Verification items for the finished model (mm, model axes). Give positions to 0.01 mm unless a question says otherwise; leave off trailing zeros. Write each loop counter-clockwise with the first axis right and the second up, starting at its lowest first coordinate (ties: lowest second). Pieces come first, ordered by that corner, then holes. Notation, with made-up numbers: (62, -23) - (83, -23) arc R21 ccw to (83, -6) - close; hole circle Ø10 at (32.25, 76). An arc over 180 degrees is marked (long way). Put each result on its own line as item: value.
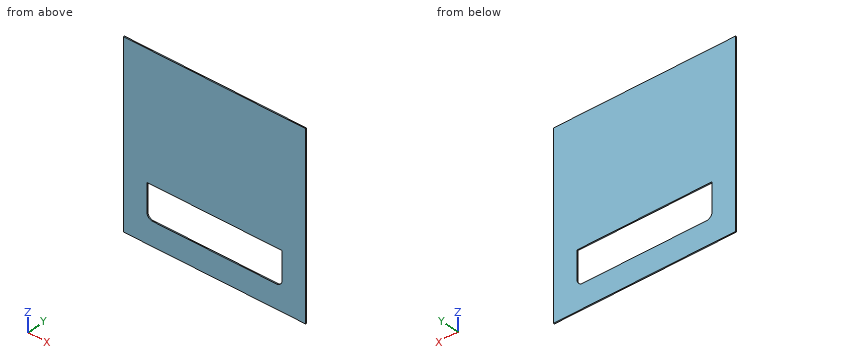
from build123d import *

# Parameters (mm, degrees)
SKETCH_1_W          = 162
SKETCH_1_H          = 162
EXTRUDE_1_DEPTH     = 1
CUT_EXTRUDE_1_REACH = 3
SKETCH_2_W          = 120
SKETCH_2_H          = 30
FILLET_1_R          = 5


with BuildPart() as part:
    # 草图1 → 凸台-拉伸1 (new body)
    with BuildSketch(Plane(origin=(0, 0, 0), x_dir=(1, 0, 0), z_dir=(0, 1, 0))):
        Rectangle(SKETCH_1_W, SKETCH_1_H)
    extrude(amount=EXTRUDE_1_DEPTH)

    # 草图2 → 切除-拉伸1 (cut, up to next)
    with BuildSketch(Plane.XZ, mode=Mode.PRIVATE) as cut_extrude_1_sk1:
        with Locations((0, -45)):
            Rectangle(SKETCH_2_W, SKETCH_2_H)
    cut_extrude_1_tool1 = extrude(cut_extrude_1_sk1.sketch, amount=-CUT_EXTRUDE_1_REACH, mode=Mode.PRIVATE) & part.part
    add(cut_extrude_1_tool1.solids().sort_by_distance((0, 0, -45))[0], mode=Mode.SUBTRACT)

    # 圆角1
    fillet_1_edges = [part.edges().sort_by_distance(p)[0] for p in [
        (60, 0.5, -60),
        (-60, 0.5, -60),
    ]]
    fillet(fillet_1_edges, radius=FILLET_1_R)


solid = part.part
Q1. Go/stop test with a flat-tipped pin: pin 1 Ø3 at (x, z) = (54.5, 31) entering from -Y. Record where the tip stops, or that it passes through.
Answers follow:
pin 1: stops at y = 0
Q2. Section check C-C, the plane y = 0.3. Record the cut outline in (x, z).
Answers follow:
outline: (-81, -81) - (81, -81) - (81, 81) - (-81, 81) - close; hole (-60, -55) arc R5 ccw to (-55, -60) - (55, -60) arc R5 ccw to (60, -55) - (60, -30) - (-60, -30) - close
Q3. Section check A-A, the plane x = 6. Record the cut outline in (y, z).
Answers follow:
outline: (0, -81) - (1, -81) - (1, -60) - (0, -60) - close; (0, -30) - (1, -30) - (1, 81) - (0, 81) - close
Q4. Scan lines: line 1 along Z through (x, y) = (23, 0.85); line 2 along X through (y, z) = (0.9, -52); line 3 along X through (y, z) = (0.7, -56.5). Record each from-to range of solid material in increasing order.
Answers follow:
line 1: z = -81 to -60, -30 to 81
line 2: x = -81 to -60, 60 to 81
line 3: x = -81 to -59.77, 59.77 to 81
Q5. Section check B-B, the plane z = -46.5. Record the cut outline in (x, y).
Answers follow:
outline: (-81, 0) - (-60, 0) - (-60, 1) - (-81, 1) - close; (60, 0) - (81, 0) - (81, 1) - (60, 1) - close
